The listing builds one solid part. Answer for the finished solid, in the listing's coordinates (mm). Round coordinates to 2 decimals unless told otherwise and drop trailing zeros. Write each loop counter-clockwise with the first axis right and the second up, starting at its lowest first coordinate (ties: lowest second). Pieces come first, ordered by that corner, then holes.
Item 1: Find section D-D on x = 4. Give the vertices of the cut face in (y, z) (3 decimals), then the cut area to 3 significant figures.
Item 2: Find section C-C on z = 1.5. Give the number of separate pieces and of enclosed holes in the cut face, then the cut area to 3 significant figures.
Item 3: Find section A-A on x = 52. Give the vertices of the cut face in (y, z) (3 decimals), then the cut area to 3 significant figures.
Item 4: Find section B-B on y = 2.5. Give the vertices of the cut face in (x, z) (3 decimals), then the cut area to 3 significant figures.
Item 5: Find the intervals of material crossed by probe 1 along X at (y, z) = (3, 1.95); probe 2 along X at (y, z) = (1.75, 0.25); probe 3 along X at (y, z) = (5, 2.2), in increasing order.
Autodesk Inventor part; units mm, degrees
ref_plane "YZ Plane" through (0, 0, 0) normal (1, 0, 0) x (0, 1, 0)
ref_plane "XZ Plane" through (0, 0, 0) normal (0, 1, 0) x (-1, 0, 0)
ref_plane "XY Plane" through (0, 0, 0) normal (0, 0, 1) x (1, 0, 0)
sketch "Sketch1" plane through (0, 0, 0) normal (0, 0, 1) x (1, 0, 0)
  line L0 (0, 0) -> (55.7735, 0)
  line L1 (55.7735, 0) -> (55.7735, 6.175)
  line L2 (55.7735, 6.175) -> (0, 6.175)
  line L3 (0, 6.175) -> (0, 0)
  line L4 (27.8868, 6.175) -> (27.8868, 0) construction
  circle A0 centre (27.8868, 3.0875) radius 1.5
  line L5 (3.0875, 6.175) -> (3.0875, 0) construction
  line L6 (52.686, 6.175) -> (52.686, 0) construction
  circle A1 centre (3.0875, 3.0875) radius 1.5
  circle A2 centre (52.686, 3.0875) radius 1.5
  line L7 (3.0875, 3.0875) -> (0, 3.0875) construction
  line L8 (52.686, 3.0875) -> (55.7735, 3.0875) construction
  line L9 (54.1985, 3.0875) -> (54.1985, 0) construction
  dimension "d4" = 3
  dimension "d8" = 49.5986
  dimension "d10" = 6.175
extrude "Extrusion1" add sketch "Sketch1" along normal blind 3.175
fillet "Fillet1" radius 3 4 edges at (0, 6.175, 1.5875) (0, 0, 1.5875) (55.7735, 6.175, 1.5875) (55.7735, 0, 1.5875)
equation "\"d4\" = hole_size"
equation "\"d5\" = hole_size"
equation "\"arm_length\" = support_length"
properties part number "_3DPrint"
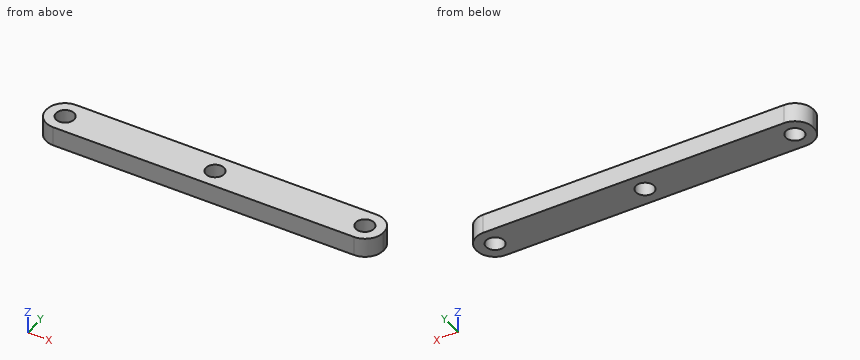
Check values:
1. outline: (0, 0) - (1.897, 0) - (1.897, 3.175) - (0, 3.175) - close; (4.278, 0) - (6.175, 0) - (6.175, 3.175) - (4.278, 3.175) - close
1. area: 12.0 mm2
2. separate pieces: 1
2. enclosed holes: 3
2. area: 315 mm2
3. outline: (0, 0) - (1.754, 0) - (1.754, 3.175) - (0, 3.175) - close; (4.421, 0) - (6.175, 0) - (6.175, 3.175) - (4.421, 3.175) - close
3. area: 11.1 mm2
4. outline: (0.042, 0) - (1.707, 0) - (1.707, 3.175) - (0.042, 3.175) - close; (4.468, 0) - (26.507, 0) - (26.507, 3.175) - (4.468, 3.175) - close; (29.267, 0) - (51.306, 0) - (51.306, 3.175) - (29.267, 3.175) - close; (54.066, 0) - (55.732, 0) - (55.732, 3.175) - (54.066, 3.175) - close
4. area: 151 mm2
5. probe 1: x = 0 to 1.59, 4.58 to 26.39, 29.38 to 51.19, 54.18 to 55.77
5. probe 2: x = 0.27 to 2.41, 3.77 to 27.21, 28.57 to 52.01, 53.37 to 55.5
5. probe 3: x = 0.62 to 55.15
